Read the model definition and answer for the solid it produces. Units are mm, in the model's axes. A direction names the side the tool comes from. Round coordinates to 2 decimals unless told otherwise and drop trailing zeros. Order: outer loops, then holes, each group sorted by start corner. A loop starts at its lowest first (then second) coordinate and runs counter-clockwise, first axis right, second up.
from build123d import *

# Parameters (mm, degrees)
F4_DEPTH  = 80
F7_DEPTH  = 30
F8_DEPTH  = 30
F9_DEPTH  = 70
F10_R     = 25
F11_DEPTH = 25
F12_R     = 20
F13_DEPTH = 30


with BuildPart() as f4:
    # F2 (on Front) → F4 (new body)
    with BuildSketch(Plane.XZ):
        with BuildLine():
            ThreePointArc((-15, 25), (-7.6776695297, 7.3223304703), (10, 0))
            Line((10, 0), (15, 0))
            Line((15, 0), (15, 105))
            ThreePointArc((15, 105), (7.6776695297, 122.6776695297), (-10, 130))
            Line((-10, 130), (-15, 130))
            Line((-15, 130), (-15, 25))
        make_face()
    extrude(amount=F4_DEPTH)

    # F3 (on Right) → F7 (join)
    with BuildSketch(Plane.YZ):
        with BuildLine():
            ThreePointArc((-51.4712392712, 67.720221312), (-40.1317472353, 65.0673444738), (-28.8207664845, 67.8392661183))
            ThreePointArc((-28.8207664845, 67.8392661183), (-40.1576697714, 69.9995856679), (-51.4712392712, 67.720221312))
        make_face()
        with BuildLine():
            ThreePointArc((-51.4712392712, 67.720221312), (-56.6712750242, 15.0586971257), (-10, 40))
            ThreePointArc((-10, 40), (-15.1466601292, 56.8021277601), (-28.8207664845, 67.8392661183))
            ThreePointArc((-28.8207664845, 67.8392661183), (-40.1317472353, 65.0673444738), (-51.4712392712, 67.720221312))
        make_face()
    extrude(amount=F7_DEPTH)

    # F3 (on Right) → F8 (join)
    with BuildSketch(Plane.YZ):
        with BuildLine():
            ThreePointArc((-51.4712392712, 67.720221312), (-40.1317472353, 65.0673444738), (-28.8207664845, 67.8392661183))
            ThreePointArc((-28.8207664845, 67.8392661183), (-40.1576697714, 69.9995856679), (-51.4712392712, 67.720221312))
        make_face()
        with BuildLine():
            ThreePointArc((-51.4712392712, 67.720221312), (-40.1576697714, 69.9995856679), (-28.8207664845, 67.8392661183))
            ThreePointArc((-28.8207664845, 67.8392661183), (-18.9199980607, 77.0489214909), (-15.2631387115, 90.066999197))
            ThreePointArc((-15.2631387115, 90.066999197), (-53.3932088942, 111.3414264983), (-51.4712392712, 67.720221312))
        make_face()
    extrude(amount=-F8_DEPTH)

    # F6 (on offset) → F9 (cut)
    with BuildSketch(Plane.XZ.offset(5)):
        Polygon((9.3415956944, 10.482782498), (10, 105), (-9.4214295968, 113.332554698), (-10, 25), align=None)
    extrude(amount=F9_DEPTH, mode=Mode.SUBTRACT)

    # F10 (on face) → F11 (cut)
    with BuildSketch(Plane.YZ.offset(30)):
        with Locations((-40, 40)):
            Circle(F10_R)
    extrude(amount=-F11_DEPTH, mode=Mode.SUBTRACT)

    # F12 (on face) → F13 (cut)
    with BuildSketch(Plane(origin=(-30, 0, 0), x_dir=(0, -1, 0), z_dir=(-1, 0, 0))):
        with Locations((40.2631387115, 90.066999197)):
            Circle(F12_R)
    extrude(amount=-F13_DEPTH, mode=Mode.SUBTRACT)


solid = f4.part
Q1. Straight lines are drawn through the part: probe 1 along Z at (x, y) = (21.25, -40); probe 2 along Y at (x, z) = (9, 89); probe 3 along Y at (x, z) = (-22.5, 108). For each, find the intervals that lie inside material, in ascending order.
Outcome:
probe 1: z = 10 to 15, 65 to 70
probe 2: y = -80 to -75, -5 to 0
probe 3: y = -57.68 to -49.12, -31.41 to -22.84
Q2. For faces 5 (the face through (0, -5, 63)), 6 (the face through (20, -60, 25)), 7 (the face through (-7.871, -39.44, 7.518)), 8 (the face through (-19.85, -35.93, 70.54)), determine the directions among +Z, -Z, +X, -X, +Y, -Y from which every point of the face is accessible in a straight line to the end or side of a thin tool.
Outcome:
face 5: none
face 6: +X
face 7: -Z, -X, +Y, -Y
face 8: -X
Q3. A cutting plane is placed at B-B, the plane x = 7. Give the vertices of the cut face in (y, z), plus the area to 3 significant figures.
Outcome:
outline: (-80, 0.18) - (0, 0.18) - (0, 123.33) - (-80, 123.33) - close; hole (-75, 12.24) - (-5, 12.24) - (-5, 106.29) - (-75, 106.29) - close
area: 3,270 mm2
Q4. Flat-ended cylindrical pins translate along their axes: pin 1 (1 mm diameter, centred on y = -51, z = 60, fed in from +X); pin 2 (6 mm diameter, centred on x = 1, y = -44, fed in from -Z); pin 3 (5 mm diameter, centred on x = 21, y = -43, fed in from -Z). Find the tip coordinate at first contact, or state that the pin passes through.
Outcome:
pin 1: stops at x = -9.77
pin 2: stops at z = 0.73
pin 3: stops at z = 10
Q5. A cutting plane is placed at C-C, the plane z = 75. Give the vertices of the cut face in (x, y).
Outcome:
outline: (-30, -60.21) - (-15, -60.21) - (-15, -80) - (15, -80) - (15, 0) - (-15, 0) - (-15, -20.31) - (-30, -20.31) - (-30, -27.11) - (-9.67, -27.11) - (-9.67, -5) - (9.79, -5) - (9.79, -75) - (-9.67, -75) - (-9.67, -53.42) - (-30, -53.42) - close
Q6. For a pull along Y with two mould halves and no side action, classify faces 1 (the face through (0, -75, 63)), 2 (the face through (0, -80, 66)), 3 (the face through (-12, -39, 130)), 4 (the face through (0.425, -39.51, 109.108)) as released by +Y, released by -Y, zero draft, split by the parting line, or undercut.
Outcome:
face 1: undercut
face 2: released by -Y
face 3: zero draft
face 4: undercut
Q7. A cutting plane is placed at D-D, the plane x = -6. Give the vertices of the cut face in (y, z), plus the area to 3 significant figures.
Outcome:
outline: (-80, 5.79) - (0, 5.79) - (0, 129.68) - (-80, 129.68) - close; hole (-75, 22) - (-5, 22) - (-5, 111.86) - (-75, 111.86) - close
area: 3,620 mm2
